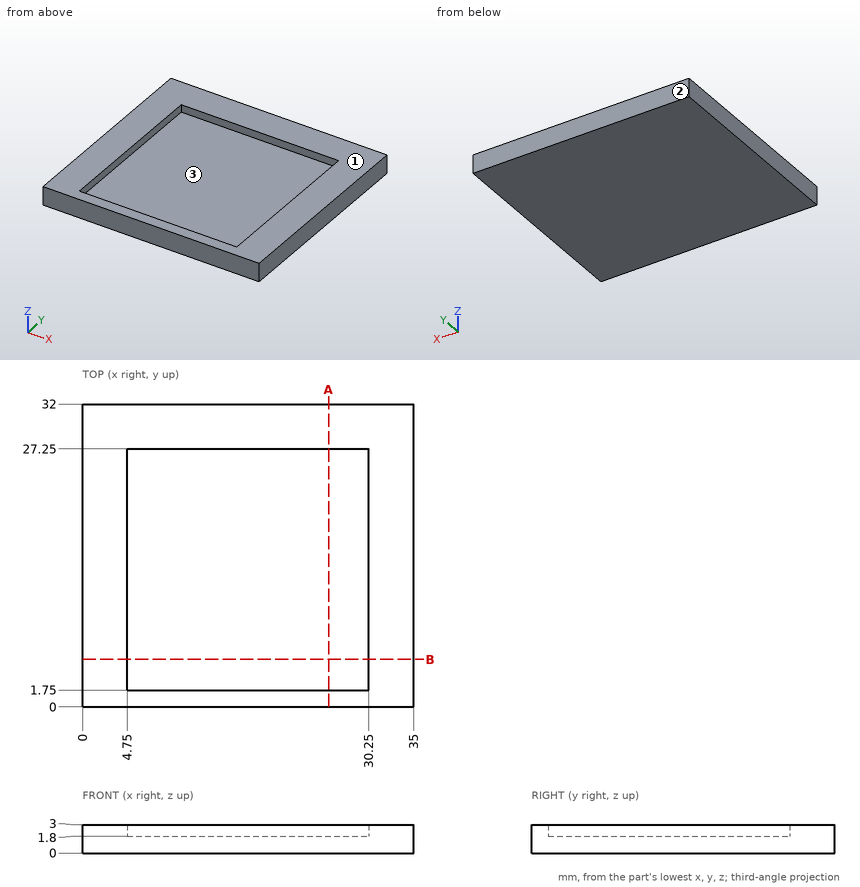
Check sheet for the drawn part. Datum: minimum x, y, z corner. Units: mm. Give positions to 0.01 mm unless a question says otherwise; leave off trailing zeros. Order: outer loops, then holes, each group sorted by start corner. A loop starts at its lowest first (then second) coordinate and runs counter-clockwise, first axis right, second up.
1. Draft check along Y on the marked faces 1, 2 and 3. Enter one of: pulls with the +Y half, pulls with the -Y half, needs draft (parallel to the pull), parting line crosses it, or undercut.
Completed:
face 1: needs draft
face 2: pulls with the +Y half
face 3: undercut
2. Depth check by flat-ended pin: pin 1 (13 mm diameter, centred on x = 20, y = 19, fed in from +Z); pin 2 (1.5 mm diameter, centred on x = 11, y = 22.5, fed in from -Z). Enter the tip coordinate at first touch or a pass-through.
Completed:
pin 1: stops at z = 1.8
pin 2: stops at z = 0
3. Scan lines: line 1 (Y direction, x = 29, z = 2.75); line 2 (X direction, y = 23.5, z = 2.6); line 3 (Z direction, x = 16, y = 22). Record each from-to range of solid material in increasing order.
Completed:
line 1: y = 0 to 1.75, 27.25 to 32
line 2: x = 0 to 4.75, 30.25 to 35
line 3: z = 0 to 1.8
4. Sectioned sample at A-A (x = 26). Record the boundary of the cut face in (y, z).
Completed:
outline: (0, 0) - (32, 0) - (32, 3) - (27.25, 3) - (27.25, 1.8) - (1.75, 1.8) - (1.75, 3) - (0, 3) - close
5. Sectioned sample at B-B (y = 5). Record the boundary of the cut face in (x, z).
Completed:
outline: (0, 0) - (35, 0) - (35, 3) - (30.25, 3) - (30.25, 1.8) - (4.75, 1.8) - (4.75, 3) - (0, 3) - close
